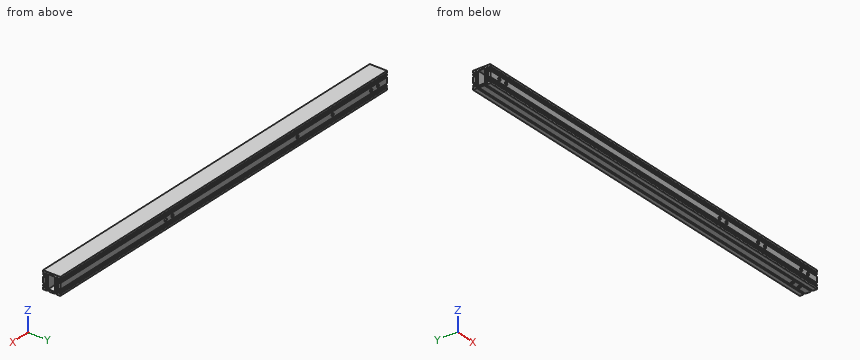
from build123d import *

# Parameters (mm, degrees)
SKETCH_1_W             = 23.5
SKETCH_1_H             = 12
EXTRUDE_1_DEPTH        = 361
HOLE_WIZARD_M6_1_D     = 5
HOLE_WIZARD_M6_1_DEPTH = 19
HOLE_WIZARD_M6_1_TIP   = 1.502151548
HOLE_WIZARD_M6_2_D     = 5
HOLE_WIZARD_M6_2_DEPTH = 19
HOLE_WIZARD_M6_2_TIP   = 1.502151548
HOLE_WIZARD_M6_3_D     = 5
HOLE_WIZARD_M6_3_DEPTH = 19
HOLE_WIZARD_M6_3_TIP   = 1.502151548


with BuildPart() as part:
    # 草图1 → 凸台-拉伸1 (new, symmetric)
    with BuildSketch(Plane(origin=(0, 0, 0), x_dir=(0, 0, -1), z_dir=(1, 0, 0))):
        Polygon((-15, 15), (-11.5, 15), (-11.5, 13.5), (-11, 13.5), (-11, 12), (-9.5, 12), (-9.5, 15), (-8, 15), (-8, 12.5), (-5, 12.5), (-5, 15), (5, 15), (5, 12.5), (8, 12.5), (8, 15), (9.5, 15), (9.5, 12), (11, 12), (11, 13.5), (11.5, 13.5), (11.5, 15), (15, 15), (15, 8), (12.5, 8), (12.5, 5), (15, 5), (15, -5), (12.5, -5), (12.5, -8), (15, -8), (15, -15), (11.5, -15), (11.5, -13.5), (11, -13.5), (11, -12), (9.5, -12), (9.5, -15), (8, -15), (8, -12.5), (5, -12.5), (5, -15), (-5, -15), (-5, -12.5), (-8, -12.5), (-8, -15), (-9.5, -15), (-9.5, -12), (-11, -12), (-11, -13.5), (-11.5, -13.5), (-11.5, -15), (-15, -15), align=None)
        with BuildLine():
            Line((12, -10.5), (12, -8.5))
            ThreePointArc((12, -8.5), (11.853553391, -8.146446609), (11.5, -8))
            Line((11.5, -8), (-11.5, -8))
            ThreePointArc((-11.5, -8), (-11.853553391, -8.146446609), (-12, -8.5))
            Line((-12, -8.5), (-12, -10.5))
            ThreePointArc((-12, -10.5), (-11.853553391, -10.853553391), (-11.5, -11))
            Line((-11.5, -11), (11.5, -11))
            ThreePointArc((11.5, -11), (11.853553391, -10.853553391), (12, -10.5))
        make_face(mode=Mode.SUBTRACT)
        with BuildLine():
            Line((-11.5, 11), (11.5, 11))
            ThreePointArc((11.5, 11), (11.853553391, 10.853553391), (12, 10.5))
            Line((12, 10.5), (12, 8.5))
            ThreePointArc((12, 8.5), (11.853553391, 8.146446609), (11.5, 8))
            Line((11.5, 8), (-11.5, 8))
            ThreePointArc((-11.5, 8), (-11.853553391, 8.146446609), (-12, 8.5))
            Line((-12, 8.5), (-12, 10.5))
            ThreePointArc((-12, 10.5), (-11.853553391, 10.853553391), (-11.5, 11))
        make_face(mode=Mode.SUBTRACT)
        Rectangle(SKETCH_1_W, SKETCH_1_H, mode=Mode.SUBTRACT)
    extrude(amount=EXTRUDE_1_DEPTH, both=True)

    # M6 螺纹孔1
    with Locations(Plane(origin=(0, -15, 0), x_dir=(-1, 0, 0), z_dir=(0, -1, 0))):
        with Locations((-341, 0), (-326, 0), (-246, 0), (-231, 0), (-161, 0), (-146, 0), (326, 0), (341, 0)):
            Hole(HOLE_WIZARD_M6_1_D / 2, depth=HOLE_WIZARD_M6_1_DEPTH)
            with Locations((0, 0, -(HOLE_WIZARD_M6_1_DEPTH + HOLE_WIZARD_M6_1_TIP / 2))):  # 118° drill point
                Cone(0, HOLE_WIZARD_M6_1_D / 2, HOLE_WIZARD_M6_1_TIP, mode=Mode.SUBTRACT)

    # M6 螺纹孔2
    with Locations(Plane(origin=(0, 15, 0), x_dir=(1, 0, 0), z_dir=(0, 1, 0))):
        with Locations((128, 0), (113, 0), (-341, 0), (-326, 0), (-241, 0), (-163, 0)):
            Hole(HOLE_WIZARD_M6_2_D / 2, depth=HOLE_WIZARD_M6_2_DEPTH)
            with Locations((0, 0, -(HOLE_WIZARD_M6_2_DEPTH + HOLE_WIZARD_M6_2_TIP / 2))):  # 118° drill point
                Cone(0, HOLE_WIZARD_M6_2_D / 2, HOLE_WIZARD_M6_2_TIP, mode=Mode.SUBTRACT)

    # M6 螺纹孔3
    with Locations(Plane(origin=(0, 0, -15), x_dir=(-1, 0, 0), z_dir=(0, 0, -1))):
        with Locations((-326, 0), (-341, 0)):
            Hole(HOLE_WIZARD_M6_3_D / 2, depth=HOLE_WIZARD_M6_3_DEPTH)
            with Locations((0, 0, -(HOLE_WIZARD_M6_3_DEPTH + HOLE_WIZARD_M6_3_TIP / 2))):  # 118° drill point
                Cone(0, HOLE_WIZARD_M6_3_D / 2, HOLE_WIZARD_M6_3_TIP, mode=Mode.SUBTRACT)


solid = part.part
Can you work these out from the model? Positions are in its coordinate system, mm. Round coordinates to 2 decimals unless told otherwise and drop trailing zeros. One line per question, with ' | ' between items. Start each with the question number.
1) I need wall thicknesses on line 1 (Y direction, x = 54, z = -9.75); line 2 (Y direction, x = 206, z = 9); line 3 (Z direction, x = 146, y = -12.3). Which ranges of each line are inside material? Lowest first, please. Write a range as [from, to].
2) Suppose I cut it at A-A on x = 27. Count the separate pieces of the cut face and the enclosed holes in it, then the cut area to 3 significant figures.
3) I'm going to push flat-ended pins straight in: P1, Ø3, axis at x = 131, z = -6, coming from the -Y side; P2, Ø4.5, axis at x = 113, z = 0, coming from the +Y side. Where does each tip first touch, or does it pass through?
Return value:
1) line 1: y = [-12, -11], [-8, -6], [6, 8], [11, 12] | line 2: y = [-15, -11], [-8, -6], [6, 8], [11, 15] | line 3: z = [-15, -11], [-9.5, -2.5], [2.5, 9.5], [11, 15]
2) separate pieces: 1 | enclosed holes: 3 | area: 408 mm2
3) P1: stops at y = -15 | P2: stops at y = -6
